from build123d import *

# Parameters (mm, degrees)
BASE_FLANGE1_DEPTH                            = 84.1502
CSK_FOR_8_FLAT_HEAD_MACHINE_SCREW1_AT_2_COUNT = 2
CSK_FOR_8_FLAT_HEAD_MACHINE_SCREW1_AT_2_PITCH = 34.925
CSK_FOR_8_FLAT_HEAD_MACHINE_SCREW2_AT_2_COUNT = 2
CSK_FOR_8_FLAT_HEAD_MACHINE_SCREW2_AT_2_PITCH = 38.1
CSK_FOR_8_FLAT_HEAD_MACHINE_SCREW3_AT_2_COUNT = 2
CSK_FOR_8_FLAT_HEAD_MACHINE_SCREW3_AT_2_PITCH = 63.5
SKETCH13_W                                    = 37.425471778
SKETCH13_H                                    = 23.818222608
CUT_EXTRUDE2_DEPTH                            = 7.62
CUT_EXTRUDE3_DEPTH                            = 31.75


# Read off the part's stored shape, not the designer's step: Base-Flange1
with BuildPart() as part:
    # Base-Flange1 outline → Base-Flange1 (new body)
    with BuildSketch(Plane.XY):
        with BuildLine():
            Line((-0.293293937, 139.7), (-6.35, 139.7))
            Line((-6.35, 139.7), (-6.35, 137.414))
            Line((-6.35, 137.414), (-0.293293937, 137.414))
            ThreePointArc((-0.293293937, 137.414), (1.103706063, 137.788325022), (2.126381041, 138.811))
            Line((2.126381041, 138.811), (2.492998462, 139.446))
            ThreePointArc((2.492998462, 139.446), (2.678939367, 139.631940905), (2.932939367, 139.7))
            Line((2.932939367, 139.7), (62.784570335, 139.7))
            ThreePointArc((62.784570335, 139.7), (63.44554116, 139.568524729), (64.005885168, 139.194114832))
            Line((64.005885168, 139.194114832), (139.194114832, 64.005885168))
            ThreePointArc((139.194114832, 64.005885168), (139.568524729, 63.44554116), (139.7, 62.784570335))
            Line((139.7, 62.784570335), (139.7, -25.4))
            Line((139.7, -25.4), (141.986, -25.4))
            Line((141.986, -25.4), (141.986, 62.784570335))
            ThreePointArc((141.986, 62.784570335), (141.68051334, 64.320355486), (140.810560934, 65.622331269))
            Line((140.810560934, 65.622331269), (65.622331269, 140.810560934))
            ThreePointArc((65.622331269, 140.810560934), (64.320355486, 141.68051334), (62.784570335, 141.986))
            Line((62.784570335, 141.986), (2.932939367, 141.986))
            ThreePointArc((2.932939367, 141.986), (1.535939367, 141.611674978), (0.513264389, 140.589))
            Line((0.513264389, 140.589), (0.146646968, 139.954))
            ThreePointArc((0.146646968, 139.954), (-0.039293937, 139.768059095), (-0.293293937, 139.7))
        make_face()
    extrude(amount=BASE_FLANGE1_DEPTH)

    # Sketch2 → CSK for #8 Flat Head Machine Screw1 (revolve, cut)
    with BuildSketch(Plane(origin=(141.986, -17.4498, 57.9501), x_dir=(0, 0, -1), z_dir=(0, 1, 0))):
        Polygon((0, 0), (0, 2.286), (2.7051, 2.286), (2.7051, 1.738551774), (4.2164, 0), align=None)
    csk_for_8_flat_head_machine_screw1 = revolve(axis=Axis((148.336, -17.4498, 57.9501), (-1, 0, 0)), mode=Mode.SUBTRACT)

    # CSK for #8 Flat Head Machine Screw1 at 2: CSK for #8 Flat Head Machine Screw1 ×2
    with Locations(*[(0, 0, -i * CSK_FOR_8_FLAT_HEAD_MACHINE_SCREW1_AT_2_PITCH) for i in range(1, CSK_FOR_8_FLAT_HEAD_MACHINE_SCREW1_AT_2_COUNT)]):
        add(csk_for_8_flat_head_machine_screw1, mode=Mode.SUBTRACT)

    # Sketch6 → CSK for #8 Flat Head Machine Screw2 (revolve, cut)
    with BuildSketch(Plane(origin=(141.986, 0, 76.2), x_dir=(0, 0, -1), z_dir=(0, 1, 0))):
        Polygon((0, 0), (0, 2.286), (2.7051, 2.286), (2.7051, 1.738551774), (4.2164, 0), align=None)
    csk_for_8_flat_head_machine_screw2 = revolve(axis=Axis((148.336, 0, 76.2), (-1, 0, 0)), mode=Mode.SUBTRACT)

    # CSK for #8 Flat Head Machine Screw2 at 2: CSK for #8 Flat Head Machine Screw2 ×2
    with Locations(*[(0, i * CSK_FOR_8_FLAT_HEAD_MACHINE_SCREW2_AT_2_PITCH, 0) for i in range(1, CSK_FOR_8_FLAT_HEAD_MACHINE_SCREW2_AT_2_COUNT)]):
        add(csk_for_8_flat_head_machine_screw2, mode=Mode.SUBTRACT)

    # Sketch8 → CSK for #8 Flat Head Machine Screw3 (revolve, cut)
    with BuildSketch(Plane(origin=(125.672839939, 80.760052265, 76.2), x_dir=(-0.707106781186544, 0.7071067811865511, 0), z_dir=(0, 0, 1))):
        Polygon((0, 0), (0, 2.286), (2.7051, 2.286), (2.7051, 1.738551774), (4.2164, 0), align=None)
    csk_for_8_flat_head_machine_screw3 = revolve(axis=Axis((130.162967999, 85.250180325, 76.2), (-0.707106781186551, -0.707106781186544, 0)), mode=Mode.SUBTRACT)

    # CSK for #8 Flat Head Machine Screw3 at 2: CSK for #8 Flat Head Machine Screw3 ×2
    with Locations(*[Vector(-0.707106781186544, 0.707106781186551, 0) * (i * CSK_FOR_8_FLAT_HEAD_MACHINE_SCREW3_AT_2_PITCH) for i in range(1, CSK_FOR_8_FLAT_HEAD_MACHINE_SCREW3_AT_2_COUNT)]):
        add(csk_for_8_flat_head_machine_screw3, mode=Mode.SUBTRACT)

    # Sketch10 → CSK for #8 Flat Head Machine Screw4 (revolve, cut)
    with BuildSketch(Plane(origin=(31.75, 141.986, 76.2), x_dir=(0, 0, 1), z_dir=(1, 0, 0))):
        Polygon((0, 0), (0, 2.286), (2.7051, 2.286), (2.7051, 1.738551774), (4.2164, 0), align=None)
    revolve(axis=Axis((31.75, 148.336, 76.2), (0, -1, 0)), mode=Mode.SUBTRACT)

    # Sketch13 → Cut-Extrude2 (cut)
    with BuildSketch(Plane(origin=(0, 141.986, 0), x_dir=(1, 0, 0), z_dir=(0, 1, 0))):
        with Locations((-15.537735889, 8.734111304)):
            Rectangle(SKETCH13_W, SKETCH13_H)
    extrude(amount=-CUT_EXTRUDE2_DEPTH, mode=Mode.SUBTRACT)

    # Sketch14 → Cut-Extrude3 (cut)
    with BuildSketch(Plane.XZ.offset(25.4)):
        Polygon((148.11255662, 7.890869199), (135.614154543, -4.139010601), (148.11255662, -4.61665654), align=None)
    extrude(amount=-CUT_EXTRUDE3_DEPTH, mode=Mode.SUBTRACT)


solid = part.part
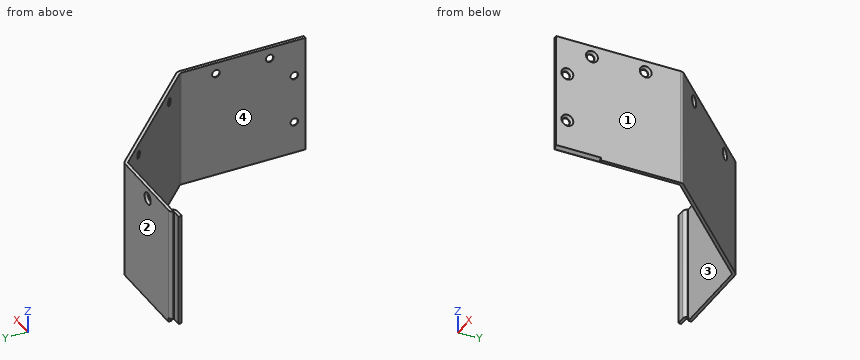
For this review, take the finished solid that the model builds, in its own axes (mm). Face numbers are marked on the shaded views. Round coordinates to 2 decimals unless told otherwise and drop trailing zeros. Order: outer loops, then holes, each group sorted by start corner. A loop starts at its lowest first (then second) coordinate and runs counter-clockwise, first axis right, second up. Notation, with made-up numbers: M 37,23.5 L 76,23.5 A19 cw 76,29.5 Z; hole C -11,-10 d3. An arc over 180 degrees is marked long. Use a Markdown table: item, result. Add a question column.
Item 1: Insertion check: pin 1 (6.5 mm diameter, centred on x = -3.5, z = 29.5, fed in from +Y); pin 2 (4.5 mm diameter, centred on x = 31.75, z = 76.2, fed in from -Y); pin 3 (5 mm diameter, centred on x = 113.5, z = 24, fed in from +Y); pin 4 (4 mm diameter, centred on x = 96.5, z = 57, fed in from +Y). Each pin has a flat end and moves straight along its axis. Give the tip position at first contact, or say it passes through.
Item 2: Add section B-B, the plane y = 0. Give the boundary of the cut face in (x, z).
Item 3: Add section A-A, the plane x = 31.75. Give the boundary of the cut face in (y, z).
Item 4: Add section C-C, the plane z = 15.5. Give the boundary of the cut face in (x, y).
Item 5: To check wall thickness, follow line 1 along Y through (x, z) = (140.15, 76.2); line 2 along Y through (x, z) = (140, 76); line 3 along Z through (x, y) = (139.8, 38.1). State the ranges of each line that lie inside material, in increasing order.
Item 6: Mouldability with a two-part tool opening along X and no side actions: class the marked faces 1, 2, 3 and 4 as released by +X, released by -X, zero draft, split by the parting line, or undercut.
Geometry results:
| question | item | result |
|---|---|---|
| 1 | pin 1 | stops at y = 139.7 |
| 1 | pin 2 | passes through |
| 1 | pin 3 | stops at y = 95.43 |
| 1 | pin 4 | stops at y = 111.93 |
| 2 | outline | M 139.7,0 L 139.91,0 L 141.99,1.99 L 141.99,71.98 L 140.25,73.49 L 139.7,73.49 Z; M 139.7,78.91 L 140.25,78.91 L 141.99,80.42 L 141.99,84.15 L 139.7,84.15 Z |
| 3 | outline | M 139.7,0 L 141.99,0 L 141.99,71.98 L 140.25,73.49 L 139.7,73.49 Z; M 139.7,78.91 L 140.25,78.91 L 141.99,80.42 L 141.99,84.15 L 139.7,84.15 Z |
| 4 | outline | M -6.35,137.41 L -0.29,137.41 A2.79 ccw 2.13,138.81 L 2.49,139.45 A0.51 cw 2.93,139.7 L 62.78,139.7 A1.73 cw 64.01,139.19 L 139.19,64.01 A1.73 cw 139.7,62.78 L 139.7,-25.4 L 141.99,-25.4 L 141.99,62.78 A4.01 ccw 140.81,65.62 L 65.62,140.81 A4.01 ccw 62.78,141.99 L 2.93,141.99 A2.79 ccw 0.51,140.59 L 0.15,139.95 A0.51 cw -0.29,139.7 L -6.35,139.7 Z |
| 5 | line 1 | y = -25.4 to -2.71, 2.71 to 35.39, 40.81 to 66.28 |
| 5 | line 2 | y = -25.4 to -2.7, 2.7 to 35.4, 40.8 to 66.43 |
| 5 | line 3 | z = 0 to 73.49, 78.91 to 84.15 |
| 6 | face 1 | released by +X |
| 6 | face 2 | zero draft |
| 6 | face 3 | undercut |
| 6 | face 4 | released by -X |
